Check sheet for the modelled part. Datum: model origin and axes. Units: mm. Face numbers are marked on the shaded views. A direction names the side the tool comes from. Give positions to 0.01 mm unless a question says otherwise; leave off trailing zeros. Write each loop counter-clockwise with the first axis right and the second up, starting at its lowest first coordinate (ties: lowest second). Pieces come first, ordered by that corner, then holes. Notation, with made-up numbers: M -12.75,35 L 32.25,35 A12 ccw 32.25,55 Z; hole C -24.75,77.5 d11. An arc over 180 degrees is marked long. Use CSV: the item, a comma, the result in double quotes. Start each with the question number.
1. Cross-section at D-D, the plane x = 11.5. Enter the section's corners in (y, z).
2. Depth check by flat-ended pin: P1, Ø3, axis at y = 2, z = -4, coming from the +X side; P2, Ø12, axis at x = 12.5, z = -31, coming from the -Y side; P3, Ø3, axis at y = 4, z = 3.5, coming from the -X side. Enter the tip coordinate at first touch or a pass-through.
3. Access from +Z, -Z, +X, -X, +Y, -Y to the whole of each face (thin tool, end or side, straight path). Record for the marked faces 1, 2 and 3.
4. Scan lines: line 1 (X direction, y = 9.5, z = 6.5); line 2 (X direction, y = 3.25, z = 16.5); line 3 (Y direction, x = 35, z = 4). Record each from-to range of solid material in increasing order.
5. Mould release check, pull along Z, two halves, no side actions. Record for the marked faces 4, 5 and 6: +Z half, -Z half, draft (parallel to the pull), parting line (faces both ways), or undercut.
6. Cross-section at B-B, the plane y = 6. Enter the section's corners in (x, z).
7. Cross-section at A-A, the plane z = 12. Enter the section's corners in (x, y), and give its area (3 significant figures).
8. Cross-section at C-C, the plane y = 2. Enter the section's corners in (x, z), and give its area (3 significant figures).
from build123d import *

# Parameters (mm, degrees)
SKETCH1_W           = 80
SKETCH1_H           = 80
BOSS_EXTRUDE1_DEPTH = 10
SKETCH2_W           = 8
SKETCH2_H           = 70
CUT_EXTRUDE1_DEPTH  = 20
CUT_EXTRUDE17_DEPTH = 75
BOSS_EXTRUDE2_DEPTH = 5
FILLET1_R           = 15


with BuildPart() as part:
    # Sketch1 → Boss-Extrude1 (new body)
    with BuildSketch(Plane(origin=(0, 0, 0), x_dir=(1, 0, 0), z_dir=(0, 1, 0))):
        Rectangle(SKETCH1_W, SKETCH1_H)
    extrude(amount=BOSS_EXTRUDE1_DEPTH)

    # Sketch2 → Cut-Extrude1 (cut)
    with BuildSketch(Plane.XZ):
        Rectangle(SKETCH2_W, SKETCH2_H)
    extrude(amount=-CUT_EXTRUDE1_DEPTH, mode=Mode.SUBTRACT)

    # Sketch8 → Cut-Extrude17 (cut)
    with BuildSketch(Plane(origin=(0, 0, -40), x_dir=(-1, 0, 0), z_dir=(0, 0, -1))):
        Polygon((-19, 0), (-22.639702343, 10), (-12.639702343, 10), (-9, 0), align=None)
    extrude(amount=-CUT_EXTRUDE17_DEPTH, mode=Mode.SUBTRACT)

    # Sketch10 → Boss-Extrude2 (add)
    with BuildSketch(Plane(origin=(0, 0, -40), x_dir=(-1, 0, 0), z_dir=(0, 0, -1))):
        Polygon((-9, 0), (-12.639702343, 10), (-22.639702343, 10), (-19, 0), align=None)
    extrude(amount=-BOSS_EXTRUDE2_DEPTH)

    # Fillet1
    # the kernel refuses this fillet: 15 mm, written as the material it takes off along each edge
    with BuildSketch(Plane(origin=(-40, 0, 75.355339059), x_dir=(1, 0, 0), z_dir=(0, 0, -1)), Plane(origin=(40, 0, -75.355339059), x_dir=(-1, 0, 0), z_dir=(0, 0, 1))) as fillet1_piece_1:
        with BuildLine():
            CenterArc((14.142135624, -15), FILLET1_R, 90, 70.528779366)
            Line((0, -10), (-0.282842712, -9.9))
            ThreePointArc((-0.282842712, -9.9), (-0.3, -5), (-0.3, 0))
            Line((-0.3, 0), (0, 0.3))
            Line((0, 0.3), (14.142135624, 0.3))
            Line((14.142135624, 0.3), (14.142135624, 0))
        make_face()
    extrude(amount=150.710678119, mode=Mode.SUBTRACT)
    with BuildSketch(Plane(origin=(-75.355339059, 0, -40), x_dir=(0, 1, 0), z_dir=(1, 0, 0)), Plane(origin=(75.355339059, 0, 40), x_dir=(0, 1, 0), z_dir=(-1, 0, 0))) as fillet1_piece_2:
        with BuildLine():
            CenterArc((15, 14.142135624), FILLET1_R, 180, 70.528779366)
            Line((0, 14.142135624), (-0.3, 14.142135624))
            Line((-0.3, 14.142135624), (-0.3, 0))
            Line((-0.3, 0), (0, -0.3))
            ThreePointArc((0, -0.3), (5, -0.3), (9.9, -0.282842712))
            Line((9.9, -0.282842712), (10, 0))
        make_face()
    extrude(amount=150.710678119, mode=Mode.SUBTRACT)


solid = part.part
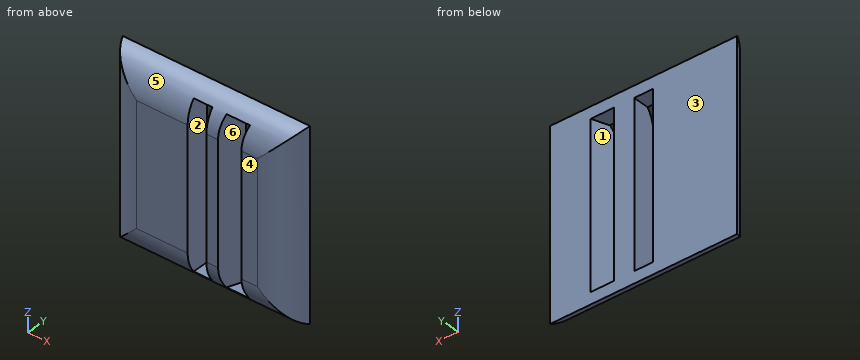
Worked answers:
1,outline,"M 3.11,-35 A15 ccw 10,-40 L 10,40 A15 ccw 3.11,35 L 6.87,35 L 6.87,-35 Z"
2,P1,"stops at x = 35.49"
2,P2,"stops at y = 0"
2,P3,"stops at x = -37.47"
3,face 1,"+Y"
3,face 2,"+Y, -Y"
3,face 3,"+Z, -Z, +X, -X, +Y"
4,line 1,"x = -39.81 to -4, 4 to 12.46, 22.46 to 39.81"
4,line 2,"x = -35.18 to -4, 4 to 10.18, 20.18 to 35.18"
4,line 3,"y = 3.11 to 10"
5,face 4,"draft"
5,face 5,"+Z half"
5,face 6,"undercut"
6,outline,"M -37.86,-37.86 L 37.86,-37.86 L 37.86,37.86 L -37.86,37.86 Z; hole M -4,-35 L 4,-35 L 4,35 L -4,35 Z; hole M 11.18,-35 L 21.18,-35 L 21.18,35 L 11.18,35 Z"
7,outline,"M -40,10 A15 ccw -25.86,0 L -4,0 L -4,10 Z; M 4,0 L 9,0 L 12.64,10 L 4,10 Z; M 19,0 L 25.86,0 A15 ccw 40,10 L 22.64,10 Z"
7,area,"543 mm^2"
8,outline,"M -33.34,-33.34 L -4,-33.34 L -4,33.34 L -33.34,33.34 Z; M 4,-33.34 L 9.73,-33.34 L 9.73,33.34 L 4,33.34 Z; M 19.73,-33.34 L 33.34,-33.34 L 33.34,33.34 L 19.73,33.34 Z"
8,area,"3,250 mm^2"
